Check sheet for the modelled part. Datum: model origin and axes. Units: mm. Round coordinates to 2 decimals unless told otherwise and drop trailing zeros. Loops run counter-clockwise (first coordinate to the right, second up) from the corner with the lowest first, then second, coordinate; pieces in that order, holes last. Notation, with made-up numbers: M -25.75,5 L -10.75,5 A18 cw -10.75,18 Z; hole C 32.25,81.5 d8. An arc over 180 degrees is marked long. Write item = value, one per line. Start each with the question number.
(1) Cross-section at C-C on y = 7. Record the boundary of the cut face in (x, z), plus the area to 3 significant figures.
(2) Go/stop test with flat-tipped pins: P1, Ø1.5, axis at x = -8, z = 3, coming from the +Y side; P2, Ø2.5, axis at y = -14, z = 2, coming from the -X side; P3, Ø3, axis at x = -3.5, y = 39, coming from the -Z side. Record where each tip stops, or that it passes through.
(3) Cross-section at A-A on x = -9. State how many separate pieces and enclosed holes the cut face has, plus the area to 3 significant figures.
(4) Scan lines: L1, parallel to X at y = 11.5, z = 4.15; L2, parallel to Y at x = -3, z = 4.6. Record each from-to range of solid material in increasing order. Write a range as from..to.
from build123d import *

# Parameters (mm, degrees)
SALIENTE_EXTRUIR1_DEPTH = 5
CROQUIS3_R              = 4
CORTAR_EXTRUIR1_DEPTH   = 5


with BuildPart() as part:
    # Croquis1 → Saliente-Extruir1 (new body)
    with BuildSketch(Plane.XY):
        Polygon((-10.50310955, 63.111111111), (-10.50310955, 53.111111111), (-5.50310955, 53.111111111), (-5.50310955, 43.111111111), (-10.50310955, 43.111111111), (-10.50310955, 33.111111111), (-5.50310955, 33.111111111), (-5.50310955, 23.111111111), (-10.50310955, 23.111111111), (-10.50310955, 13.111111111), (-5.50310955, 13.111111111), (-5.50310955, 3.111111111), (-10.50310955, 3.111111111), (-10.50310955, -6.888888889), (-5.50310955, -6.888888889), (-5.50310955, -16.888888889), (-10.50310955, -16.888888889), (-10.50310955, -26.888888889), (-5.50310955, -26.888888889), (-5.50310955, -36.888888889), (-10.50310955, -36.888888889), (-10.50310955, -46.888888889), (-5.50310955, -46.888888889), (-5.50310955, -56.888888889), (-10.50310955, -56.888888889), (-10.50310955, -66.888888889), (-5.50310955, -66.888888889), (-5.50310955, -76.888888889), (-10.50310955, -76.888888889), (-10.50310955, -86.888888889), (-0.50310955, -86.888888889), (-0.50310955, 73.111111111), (-5.50310955, 73.111111111), (-5.50310955, 63.111111111), align=None)
    extrude(amount=SALIENTE_EXTRUIR1_DEPTH)

    # Croquis3 → Cortar-Extruir1 (cut)
    with BuildSketch(Plane.ZY.offset(5.50310955)):
        with Locations((6.5, 7.201111111)):
            Circle(CROQUIS3_R)
    extrude(amount=-CORTAR_EXTRUIR1_DEPTH, mode=Mode.SUBTRACT)


solid = part.part
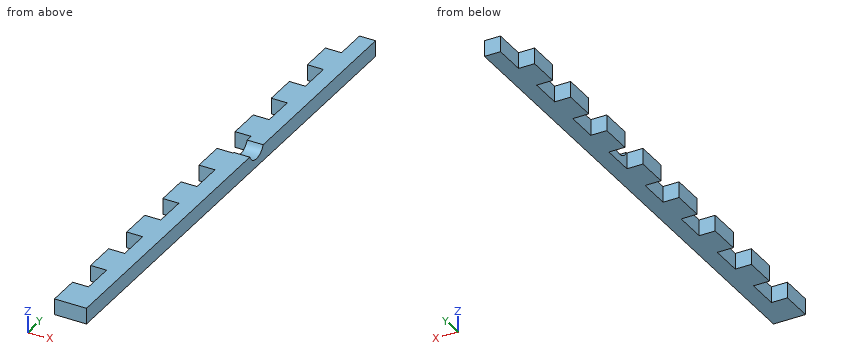
Result:
q1.outline = M -5.5,0 L -0.5,0 L -0.5,2.51 L -5.5,2.51 Z
q1.area = 12.5 mm^2
q2.P1 = 63.11
q2.P2 = -5.5
q2.P3 = 0
q3.separate_pieces = 8
q3.enclosed_holes = 0
q3.area = 400 mm^2
q4.L1 = -5.5..-0.5
q4.L2 = -86.89..3.68, 10.72..73.11
